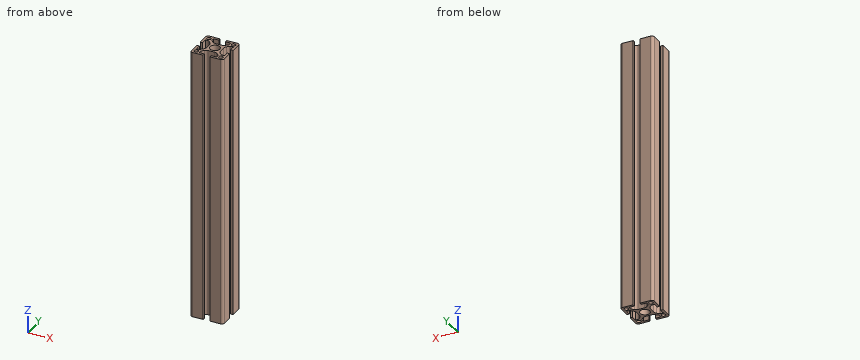
Autodesk Inventor part; units mm, degrees
ref_plane "side_4d_XY" through (-20, 0, -165) normal (-1, 0, 0) x (0, 1, 0)
ref_plane "side_4d_YZ" through (-20, 0, -165) normal (0, 1, 0) x (0, 0, -1)
ref_plane "side_4d_ZX" through (-20, 0, -165) normal (0, 0, -1) x (-1, 0, 0)
sketch "Skizze_1" plane through (0, 0, 0) normal (0, 0, 1) x (1, 0, 0)
  arc A0 (-20, -17) -> (-17, -20) centre (-17, -17) ccw
  line L0 (-17, -20) -> (-4.1, -20)
  line L1 (-4.1, -20) -> (-4.1, -17)
  line L2 (-4.1, -17) -> (-10.5, -17)
  line L3 (-10.5, -17) -> (-10.5, -13.6627)
  arc A1 (-10.0314, -12.5314) -> (-10.5, -13.6627) centre (-8.9002, -13.6627) ccw
  line L4 (-10.0314, -12.5314) -> (-7.4645, -9.9645)
  arc A2 (-3.9289, -8.5) -> (-7.4645, -9.9645) centre (-3.9289, -13.5) ccw
  line L5 (-3.9289, -8.5) -> (3.9289, -8.5)
  arc A3 (7.4645, -9.9645) -> (3.9289, -8.5) centre (3.9289, -13.5) ccw
  line L6 (7.4645, -9.9645) -> (10.0314, -12.5314)
  arc A4 (10.5, -13.6627) -> (10.0314, -12.5314) centre (8.9002, -13.6627) ccw
  line L7 (10.5, -13.6627) -> (10.5, -17)
  line L8 (10.5, -17) -> (4.1, -17)
  line L9 (4.1, -17) -> (4.1, -20)
  line L10 (4.1, -20) -> (17, -20)
  arc A5 (17, -20) -> (20, -17) centre (17, -17) ccw
  line L11 (20, -17) -> (20, -4.1)
  line L12 (20, -4.1) -> (17, -4.1)
  line L13 (17, -4.1) -> (17, -10.5)
  line L14 (17, -10.5) -> (13.6627, -10.5)
  arc A6 (12.5314, -10.0314) -> (13.6627, -10.5) centre (13.6627, -8.9002) ccw
  line L15 (12.5314, -10.0314) -> (9.9645, -7.4645)
  arc A7 (8.5, -3.9289) -> (9.9645, -7.4645) centre (13.5, -3.9289) ccw
  line L16 (8.5, -3.9289) -> (8.5, 3.9289)
  arc A8 (9.9645, 7.4645) -> (8.5, 3.9289) centre (13.5, 3.9289) ccw
  line L17 (9.9645, 7.4645) -> (12.5314, 10.0314)
  arc A9 (13.6627, 10.5) -> (12.5314, 10.0314) centre (13.6627, 8.9002) ccw
  line L18 (13.6627, 10.5) -> (17, 10.5)
  line L19 (17, 10.5) -> (17, 4.1)
  line L20 (17, 4.1) -> (20, 4.1)
  line L21 (20, 4.1) -> (20, 17)
  arc A10 (20, 17) -> (17, 20) centre (17, 17) ccw
  line L22 (17, 20) -> (4.1, 20)
  line L23 (4.1, 20) -> (4.1, 17)
  line L24 (4.1, 17) -> (10.5, 17)
  line L25 (10.5, 17) -> (10.5, 13.6627)
  arc A11 (10.0314, 12.5314) -> (10.5, 13.6627) centre (8.9002, 13.6627) ccw
  line L26 (10.0314, 12.5314) -> (7.4645, 9.9645)
  arc A12 (3.9289, 8.5) -> (7.4645, 9.9645) centre (3.9289, 13.5) ccw
  line L27 (3.9289, 8.5) -> (-3.9289, 8.5)
  arc A13 (-7.4645, 9.9645) -> (-3.9289, 8.5) centre (-3.9289, 13.5) ccw
  line L28 (-7.4645, 9.9645) -> (-10.0314, 12.5314)
  arc A14 (-10.5, 13.6627) -> (-10.0314, 12.5314) centre (-8.9002, 13.6627) ccw
  line L29 (-10.5, 13.6627) -> (-10.5, 17)
  line L30 (-10.5, 17) -> (-4.1, 17)
  line L31 (-4.1, 17) -> (-4.1, 20)
  line L32 (-4.1, 20) -> (-17, 20)
  arc A15 (-17, 20) -> (-20, 17) centre (-17, 17) ccw
  line L33 (-20, 17) -> (-20, 4.1)
  line L34 (-20, 4.1) -> (-17, 4.1)
  line L35 (-17, 4.1) -> (-17, 10.5)
  line L36 (-17, 10.5) -> (-13.6627, 10.5)
  arc A16 (-12.5314, 10.0314) -> (-13.6627, 10.5) centre (-13.6627, 8.9002) ccw
  line L37 (-12.5314, 10.0314) -> (-9.9645, 7.4645)
  arc A17 (-8.5, 3.9289) -> (-9.9645, 7.4645) centre (-13.5, 3.9289) ccw
  line L38 (-8.5, 3.9289) -> (-8.5, -3.9289)
  arc A18 (-9.9645, -7.4645) -> (-8.5, -3.9289) centre (-13.5, -3.9289) ccw
  line L39 (-9.9645, -7.4645) -> (-12.5314, -10.0314)
  arc A19 (-13.6627, -10.5) -> (-12.5314, -10.0314) centre (-13.6627, -8.9002) ccw
  line L40 (-13.6627, -10.5) -> (-17, -10.5)
  line L41 (-17, -10.5) -> (-17, -4.1)
  line L42 (-17, -4.1) -> (-20, -4.1)
  line L43 (-20, -4.1) -> (-20, -17)
  circle A20 centre (0, 0) radius 6
extrude "Extrusion1" add sketch "Skizze_1" against normal blind 330
sketch "Sketch2" plane through (0, 0, 0) normal (0, 0, 1) x (1, 0, 0)
  point P0 (-15, -15)
hole "Drilling 1" at (-15, -15, 0) direction (0, 0, -1) diameter 5 depth 6000
sketch "Sketch3" plane through (0, 0, 0) normal (0, 0, 1) x (1, 0, 0)
  point P0 (15, -15)
hole "Drilling 2" at (15, -15, 0) direction (0, 0, -1) diameter 5 depth 6000
sketch "Sketch4" plane through (0, 0, 0) normal (0, 0, 1) x (1, 0, 0)
  point P0 (15, 15)
hole "Drilling 3" at (15, 15, 0) direction (0, 0, -1) diameter 5 depth 6000
sketch "Sketch5" plane through (0, 0, 0) normal (0, 0, 1) x (1, 0, 0)
  point P0 (-15, 15)
hole "Drilling 4" at (-15, 15, 0) direction (0, 0, -1) diameter 5 depth 6000
ref_plane "side_4d_XY" through (-20, 0, -165) normal (-1, 0, 0) x (0, 1, 0)
ref_plane "side_4d_YZ" through (-20, 0, -165) normal (0, 1, 0) x (0, 0, -1)
ref_plane "side_4d_ZX" through (-20, 0, -165) normal (0, 0, -1) x (-1, 0, 0)
ref_plane "side_1a_XY" through (0, 20, -165) normal (0, 1, 0) x (1, 0, 0)
ref_plane "side_1a_YZ" through (0, 20, -165) normal (1, 0, 0) x (0, 0, -1)
ref_plane "side_1a_ZX" through (0, 20, -165) normal (0, 0, -1) x (0, 1, 0)
ref_plane "side_2b_XY" through (20, 0, -165) normal (1, 0, 0) x (0, -1, 0)
ref_plane "side_2b_YZ" through (20, 0, -165) normal (0, -1, 0) x (0, 0, -1)
ref_plane "side_2b_ZX" through (20, 0, -165) normal (0, 0, -1) x (1, 0, 0)
ref_plane "side_3c_XY" through (0, -20, -165) normal (0, -1, 0) x (-1, 0, 0)
ref_plane "side_3c_YZ" through (0, -20, -165) normal (-1, 0, 0) x (0, 0, -1)
ref_plane "side_3c_ZX" through (0, -20, -165) normal (0, 0, -1) x (0, -1, 0)
ref_plane "end_XY" through (0, 0, -330) normal (0, 0, -1) x (1, 0, 0)
ref_plane "end_YZ" through (0, 0, -330) normal (1, 0, 0) x (0, -1, 0)
ref_plane "end_ZX" through (0, 0, -330) normal (0, -1, 0) x (0, 0, -1)
ref_plane "start_XY" through (0, 0, 0) normal (0, 0, 1) x (1, 0, 0)
ref_plane "start_YZ" through (0, 0, 0) normal (1, 0, 0) x (0, 1, 0)
ref_plane "start_ZX" through (0, 0, 0) normal (0, 1, 0) x (0, 0, 1)
properties part number "MayTec 1.11.040040.43S_Profile 40x40, 4E, S_330_Detail_(0;0,0,0)"
Source: CAD feature listing. Evaluate the final solid. Frame: model axes, mm. Round coordinates to 2 decimals unless told otherwise and drop trailing zeros. Loops run counter-clockwise (first coordinate to the right, second up) from the corner with the lowest first, then second, coordinate; pieces in that order, holes last. Notation, with made-up numbers: M 70,83.5 L 80,83.5 A27 cw 80,120.5 Z; hole C 8.5,-2 d7. An arc over 180 degrees is marked long. Answer as CSV lines item,"result".
Q1. Line query: line 1 along Y through (x, z) = (8, -130); line 2 along Y through (x, z) = (-15, -242.5). Output: solid intervals per line, ascending.
Verdict:
line 1,"y = -20 to -17, -10.5 to 10.5, 17 to 20"
line 2,"y = -20 to -17.5, -12.5 to -10.5, 10.5 to 12.5, 17.5 to 20"
Q2. Cut plane A-A (y = 0). Return the cut outline in (x, z).
Verdict:
outline,"M -8.5,-330 L -6,-330 L -6,0 L -8.5,0 Z; M 6,-330 L 8.5,-330 L 8.5,0 L 6,0 Z"
Q3. Contact query for flat-ended pins moving along their axis: pin 1 (0.9 mm diameter, centred on x = 19, z = -158, fed in from -Y); pin 2 (0.9 mm diameter, centred on y = -18, z = -202.5, fed in from +X); pin 3 (1.5 mm diameter, centred on y = 19, z = -161, fed in from +X). Output: stop coordinate, or through.
Verdict:
pin 1,"stops at y = -19.57"
pin 2,"stops at x = 19.95"
pin 3,"stops at x = 19.73"
Q4. Cut plane C-C (z = -55). Count the separate pieces of the cut face and the enclosed holes in it, plus the area to 3 significant figures.
Verdict:
separate pieces,"1"
enclosed holes,"5"
area,"674 mm^2"
